Source: CAD feature listing. Evaluate the final solid. Frame: model axes, mm. A direction names the side the tool comes from. Round coordinates to 2 decimals unless told otherwise and drop trailing zeros. Loops run counter-clockwise (first coordinate to the right, second up) from the corner with the lowest first, then second, coordinate; pieces in that order, holes last.
Item 1: Ray query, L1, parallel to Z at x = 0, y = -14.25; L2, parallel to Z at x = 2.25, y = -4.5; L3, parallel to X at y = -16.5, z = 0.25. Return the intervals inside material, ascending.
Item 2: First-contact query: P1, Ø0.5, axis at x = -0.5, y = -0.5, coming from the -Z side; P2, Ø1.6, axis at x = 5, z = 0.5, coming from the +Y side; P3, Ø6, axis at x = 4.5, y = -4.5, coming from the -Z side. Flat tips, straight axial feed; report the tip coordinate or a pass-through.
Item 3: Section query B-B on y = -12.25. Return loops of the section in (x, z).
Item 4: Section query D-D on y = -8.25. Return loops of the section in (x, z).
Item 5: Pull-direction query (Z, two-part tool) for faces 1 (the flat face through (6, -20, 0)), 2 (the flat face through (0.673, -0.493, -0.096)), 3 (the flat face through (0, -0.5, 1.732)), 4 (the flat face through (6, -23, 1)); classes: released by +Z, released by -Z, zero draft, split by the parting line, or undercut.
Item 6: Section query C-C on z = 2.5. Return loops of the section in (x, y), then the cut area to 3 significant figures.
Item 7: Access query for faces 5 (the flat face through (2, -25, 2)), 6 (the flat face through (0, -10, 0)), 7 (the flat face through (0, -0.5, 2.165)), 8 (the flat face through (6, -23, -1)). Directions: +Z, -Z, +X, -X, +Y, -Y. A direction counts if a zero-diameter tool reaches every point of the face in a straight line with its end or side. Return the directions, or none.
```python
from build123d import *

# Parameters (mm, degrees)
F0_R     = 3.75
F1_DEPTH = 25
F2_W     = 8
F2_H     = 2
F3_DEPTH = 5
F4_R     = 0.99999
F5_R     = 2.1
F6_DEPTH = 15
F7_R     = 3
F7_R_2   = 2.75
F8_DEPTH = 1
F9_R     = 1


# Not quite as in the source:
# - a fillet or chamfer is up to 0.001 mm smaller than in the source, because OpenCascade refuses the exact size


with BuildPart() as f1:
    # F0 (on Front) → F1 (new body)
    with BuildSketch(Plane.XZ):
        Circle(F0_R)
    extrude(amount=F1_DEPTH)

    # F2 (on face) → F3 (join)
    with BuildSketch(Plane.XZ.offset(25)):
        with Locations((3.75, 0)):
            Rectangle(F2_W, F2_H)
    extrude(amount=-F3_DEPTH)

    # F4 (radius 1 in the source; OpenCascade refuses exactly that, so slightly less here)
    f4_edges = [f1.edges().sort_by_distance(p)[0] for p in [
        (3.614208, -22.5, 1),
        (3.614208, -22.5, -1),
        (7.75, -22.5, 1),
        (7.75, -22.5, -1),
    ]]
    fillet(f4_edges, radius=F4_R)

    # F5 (on face) → F6 (cut)
    with BuildSketch(Plane.XZ.offset(25)):
        Circle(F5_R)
    extrude(amount=-F6_DEPTH, mode=Mode.SUBTRACT)

    # F7 (on face) → F8 (cut)
    with BuildSketch(Plane(origin=(0, 0, 0), x_dir=(-1, 0, 0), z_dir=(0, 1, 0))):
        Circle(F7_R)
        Circle(F7_R_2, mode=Mode.SUBTRACT)
        Polygon((1.25, -2.1650635095), (2.5, 0), (1.25, 2.1650635095), (-1.25, 2.1650635095), (-2.5, 0), (-1.25, -2.1650635095), align=None)
        with BuildLine():
            ThreePointArc((1, 1.7320508076), (1.7320508076, 1), (2, 0))
            ThreePointArc((2, 0), (1.7320508076, -1), (1, -1.7320508076))
            ThreePointArc((1, -1.7320508076), (0, -2), (-1, -1.7320508076))
            ThreePointArc((-1, -1.7320508076), (-1.7320508076, -1), (-2, 0))
            ThreePointArc((-2, 0), (-1.7320508076, 1), (-1, 1.7320508076))
            ThreePointArc((-1, 1.7320508076), (0, 2), (1, 1.7320508076))
        make_face(mode=Mode.SUBTRACT)
        with BuildLine():
            Line((-2, 0), (-1, 1.7320508076))
            ThreePointArc((-1, 1.7320508076), (-1.7320508076, 1), (-2, 0))
        make_face()
        with BuildLine():
            Line((-1, 1.7320508076), (1, 1.7320508076))
            ThreePointArc((1, 1.7320508076), (0, 2), (-1, 1.7320508076))
        make_face()
        with BuildLine():
            ThreePointArc((-2, 0), (-1.7320508076, -1), (-1, -1.7320508076))
            Line((-1, -1.7320508076), (-2, 0))
        make_face()
        with BuildLine():
            ThreePointArc((1, -1.7320508076), (1.7320508076, -1), (2, 0))
            Line((2, 0), (1.5, -0.8660254038))
            Line((1.5, -0.8660254038), (1, -1.7320508076))
        make_face()
        with BuildLine():
            Line((1, 1.7320508076), (2, 0))
            ThreePointArc((2, 0), (1.7320508076, 1), (1, 1.7320508076))
        make_face()
        with BuildLine():
            ThreePointArc((-1, -1.7320508076), (0, -2), (1, -1.7320508076))
            Line((1, -1.7320508076), (-1, -1.7320508076))
        make_face()
        Polygon((0.8465453085, -0.7060742072), (0.8991730442, -0.4951797253), (-0.5881552807, 1.095739762), (-0.7212159254, 1.0418686678), align=None)
        Polygon((-0.7212159254, 1.0418686678), (-0.85427657, 0.9879975736), (-0.8180661444, -1.0666475449), (-0.6253293831, -1.2018198644), align=None)
        Polygon((-0.4325926219, -1.3369921838), (0.7939175728, -0.9169686891), (0.8465453085, -0.7060742072), (-0.6253293831, -1.2018198644), align=None)
        Polygon((-0.8180661444, -1.0666475449), (-0.8110177635, -1.4665854405), (-0.4325926219, -1.3369921838), (-0.6253293831, -1.2018198644), align=None)
        Polygon((0.7939175728, -0.9169686891), (1.1723427144, -0.7873754324), (0.8991730442, -0.4951797253), (0.8465453085, -0.7060742072), align=None)
        Polygon((-0.5881552807, 1.095739762), (-0.8613249509, 1.3879354691), (-0.85427657, 0.9879975736), (-0.7212159254, 1.0418686678), align=None)
    extrude(amount=-F8_DEPTH, mode=Mode.SUBTRACT)

    # F9
    f9_edges = [f1.edges().sort_by_distance(p)[0] for p in [
        (-2.1, -10, 0),
    ]]
    fillet(f9_edges, radius=F9_R)


solid = f1.part
```
Data:
1. L1: z = -3.75 to -2.1, 2.1 to 3.75
1. L2: z = -3 to 3
1. L3: x = -3.74 to -2.09, 2.09 to 3.74
2. P1: stops at z = -3.74
2. P2: stops at y = -20
2. P3: stops at z = -3.44
3. outline: circle Ø7.5 at (0, 0); hole circle Ø4.2 at (0, 0)
4. outline: circle Ø7.5 at (0, 0)
5. face 1: zero draft
5. face 2: undercut
5. face 3: undercut
5. face 4: released by +Z
6. outline: (-2.8, -25) - (2.8, -25) - (2.8, 0) - (1.66, 0) - (1.66, -1) - (1.15, -1) - (1.15, 0) - (-1.15, 0) - (-1.15, -1) - (-1.66, -1) - (-1.66, 0) - (-2.8, 0) - close
6. area: 139 mm2
7. face 5: +Z, -Z, +X, -X, -Y
7. face 6: -Y
7. face 7: +Y
7. face 8: -Z, +X, +Y, -Y
